Verification items for this drawing (mm, ordinates from the low corner). A direction names the side the tool comes from. Coordinates: 2 decimals unless noted, no trailing zeros. Write each loop counter-clockwise with the first axis right and the second up, starting at its lowest first coordinate (ties: lowest second). Pieces come first, ordered by that corner, then holes. Notation, with made-up numbers: M -8.5,38 L 20.5,38 A14 ccw 20.5,59 Z; hole C 65,45 d7. An arc over 180 degrees is marked long. Write each question's results on one line, items separated by ' | '.
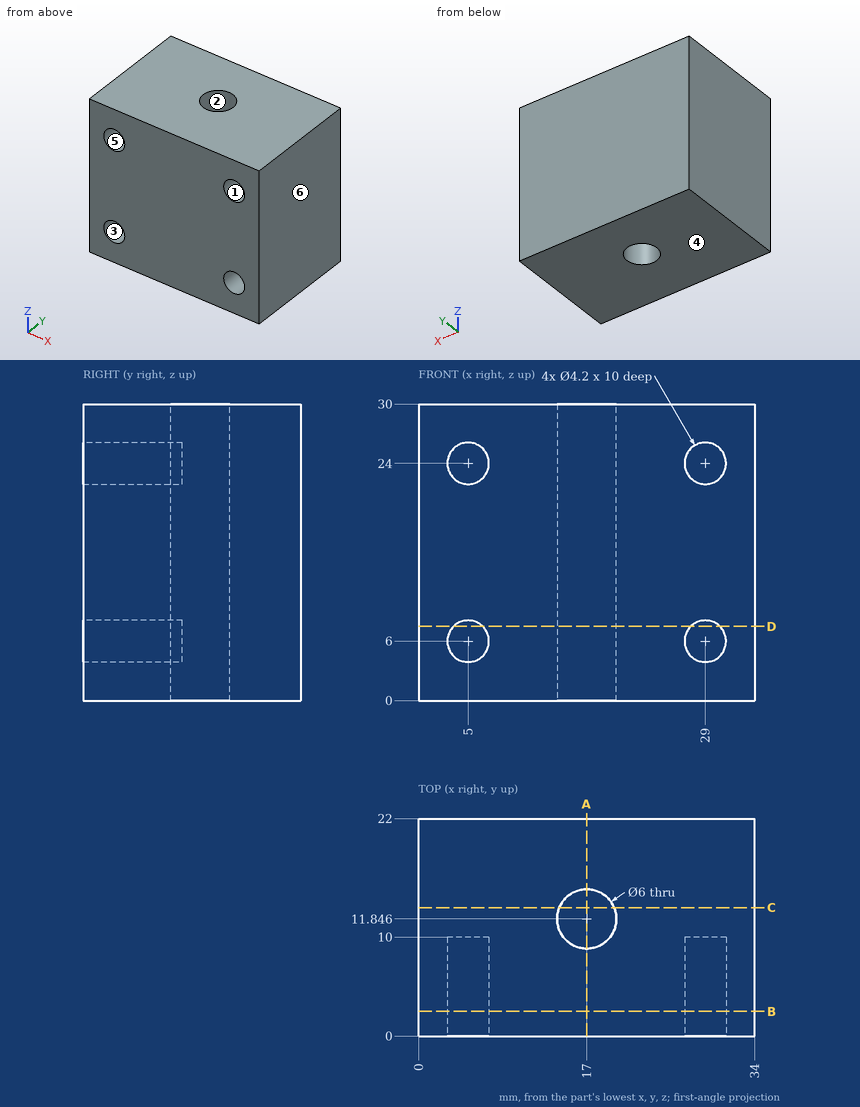
Q1. Sectioned sample at C-C on y = 13. Record the cut outline in (x, z), and give its area (3 significant figures).
Geometry check:
outline: M 0,0 L 14.23,0 L 14.23,30 L 0,30 Z; M 19.77,0 L 34,0 L 34,30 L 19.77,30 Z | area: 854 mm2
Q2. Sectioned sample at A-A on x = 17. Record the cut outline in (y, z).
Geometry check:
outline: M 0,0 L 8.85,0 L 8.85,30 L 0,30 Z; M 14.85,0 L 22,0 L 22,30 L 14.85,30 Z
Q3. Depth check by flat-ended pin: P1, Ø12, axis at x = 4, z = 21, coming from the -Y side; P2, Ø2.5, axis at x = 29, z = 6, coming from the -Y side. Enter the tip coordinate at first touch or a pass-through.
Geometry check:
P1: stops at y = 0 | P2: stops at y = 10
Q4. Sectioned sample at D-D on z = 7.5. Record the cut outline in (x, y).
Geometry check:
outline: M 0,0 L 3.53,0 L 3.53,10 L 6.47,10 L 6.47,0 L 27.53,0 L 27.53,10 L 30.47,10 L 30.47,0 L 34,0 L 34,22 L 0,22 Z; hole C 17,11.85 d6
Q5. Scan lines: probe 1 along X at (y, z) = (3.75, 6); probe 2 along Y at (x, z) = (17, 5.75); probe 3 along X at (y, z) = (5.5, 24.75). Record each from-to range of solid material in increasing order.
Geometry check:
probe 1: x = 0 to 2.9, 7.1 to 26.9, 31.1 to 34 | probe 2: y = 0 to 8.85, 14.85 to 22 | probe 3: x = 0 to 3.04, 6.96 to 27.04, 30.96 to 34
Q6. Mould release check, pull along Z, two halves, no side actions. Record for the marked faces 3, 4, 5 and 6: pulls with the +Z half, pulls with the -Z half, needs draft (parallel to the pull), parting line crosses it, or undercut.
Geometry check:
face 3: undercut | face 4: pulls with the -Z half | face 5: undercut | face 6: needs draft
Q7. Sectioned sample at B-B on y = 2.5. Record the cut outline in (x, z).
Geometry check:
outline: M 0,0 L 34,0 L 34,30 L 0,30 Z; hole C 5,6 d4.2; hole C 5,24 d4.2; hole C 29,6 d4.2; hole C 29,24 d4.2
Q8. Access from +Z, -Z, +X, -X, +Y, -Y to the whole of each face (thin tool, end or side, straight path). Record for the marked faces 1 and 2.
Geometry check:
face 1: -Y | face 2: +Z, -Z
